Check sheet for the drawn part. Datum: minimum x, y, z corner. Units: mm. A direction names the side the tool comes from. Coordinates: 2 decimals unless noted, no trailing zeros. Write each loop counter-clockwise with the first axis right and the second up, starting at its lowest first coordinate (ties: lowest second). Pieces come first, ordered by that corner, then holes. Notation, with made-up numbers: M -3,20.5 L 56,20.5 A13 ccw 56,28.5 Z; hole C 47.25,-16 d10. An arc over 180 degrees is marked long. Answer in a Markdown table with one row per item.
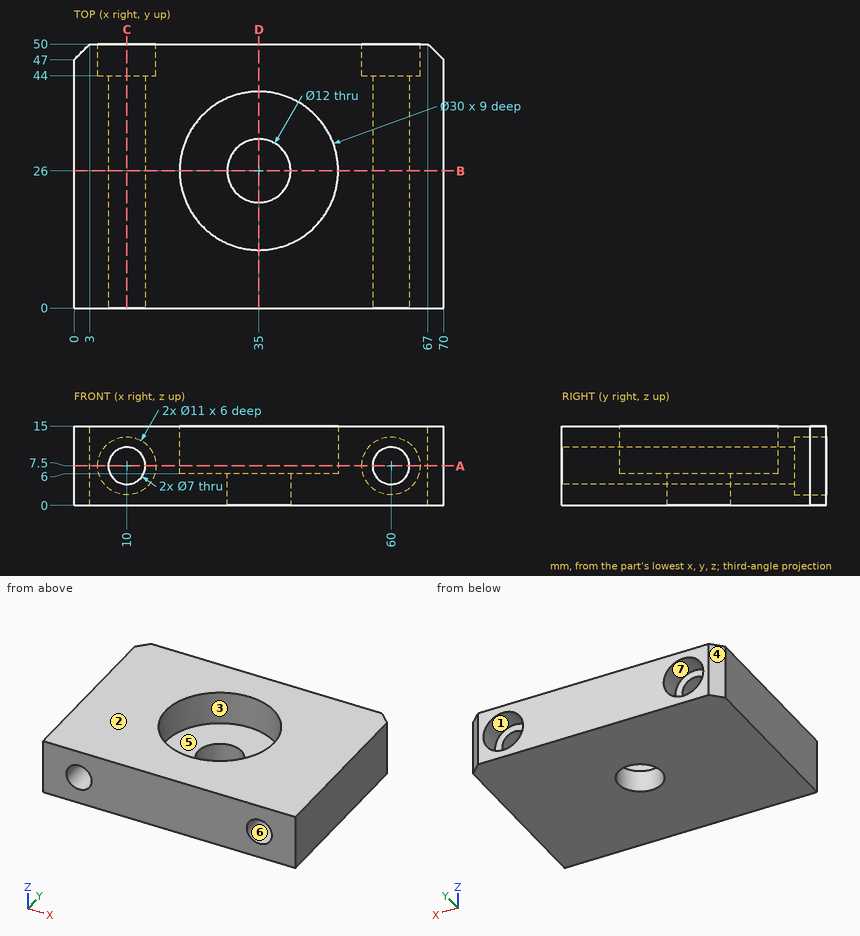
1) Depth check by flat-ended pin: pin 1 (3.5 mm diameter, centred on x = 11.5, z = 9.5, fed in from +Y); pin 2 (8 mm diameter, centred on x = 10, z = 7.5, fed in from -Y); pin 3 (3 mm diameter, centred on x = 31.5, y = 37, fed in from +Z). Enter the tip coordinate at first touch or a pass-through.
Response values:
| item | result |
|---|---|
| pin 1 | stops at y = 44 |
| pin 2 | stops at y = 0 |
| pin 3 | stops at z = 6 |
2) Thickness scan on L1, parallel to Y at x = 35, z = 10.25; L2, parallel to X at y = 22, z = 10.5; L3, parallel to Y at x = 35, z = 4.35. Record the ranges inside material, lowest first. Write a range as [from, to].
Response values:
| item | result |
|---|---|
| L1 | y = [0, 11], [41, 50] |
| L2 | x = [0, 8.2], [11.8, 20.54], [49.46, 58.2], [61.8, 70] |
| L3 | y = [0, 20], [32, 50] |
3) Sectioned sample at D-D (x = 35). Record the cut outline in (y, z).
Response values:
| item | result |
|---|---|
| outline | M 0,0 L 20,0 L 20,6 L 11,6 L 11,15 L 0,15 Z; M 32,0 L 50,0 L 50,15 L 41,15 L 41,6 L 32,6 Z |
4) Sectioned sample at A-A (z = 7.5). Record the cut outline in (x, y), then the cut area to 3 significant figures.
Response values:
| item | result |
|---|---|
| outline | M 0,0 L 6.5,0 L 6.5,44 L 4.5,44 L 4.5,50 L 3,50 L 0,47 Z; M 13.5,0 L 56.5,0 L 56.5,44 L 54.5,44 L 54.5,50 L 15.5,50 L 15.5,44 L 13.5,44 Z; M 63.5,0 L 70,0 L 70,47 L 67,50 L 65.5,50 L 65.5,44 L 63.5,44 Z; hole C 35,26 d30 |
| area | 2,040 mm² |
5) Tool access check on the marked faces 1, 2 and 3. Record the directions out of +Z, -Z, +X, -X, +Y, -Y that give a thin tool (end or side, any length) a straight path to the whole face; none if there is none.
Response values:
| item | result |
|---|---|
| face 1 | +Y |
| face 2 | +Z, +X, -X, +Y, -Y |
| face 3 | +Z |
6) Release check for a two-part mould opening along Z. For the marked faces 4, 5, 6 and 7 record: +Z half, -Z half, draft (parallel to the pull), parting line (faces both ways), or undercut.
Response values:
| item | result |
|---|---|
| face 4 | draft |
| face 5 | +Z half |
| face 6 | undercut |
| face 7 | undercut |
7) Sectioned sample at B-B (y = 26). Record the cut outline in (x, z), then the cut area to 3 significant figures.
Response values:
| item | result |
|---|---|
| outline | M 0,0 L 29,0 L 29,6 L 20,6 L 20,15 L 0,15 Z; M 41,0 L 70,0 L 70,15 L 50,15 L 50,6 L 41,6 Z; hole C 10,7.5 d7; hole C 60,7.5 d7 |
| area | 631 mm² |
8) Sectioned sample at C-C (x = 10). Record the cut outline in (y, z), then the cut area to 3 significant figures.
Response values:
| item | result |
|---|---|
| outline | M 0,0 L 50,0 L 50,2 L 44,2 L 44,4 L 0,4 Z; M 0,11 L 44,11 L 44,13 L 50,13 L 50,15 L 0,15 Z |
| area | 376 mm² |
